For this review, take the finished solid that the model builds, in its own axes (mm). Round coordinates to 2 decimals unless told otherwise and drop trailing zeros. Order: outer loops, then holes, each group sorted by start corner. A loop starts at its lowest first (then second) coordinate and runs counter-clockwise, first axis right, second up. Notation, with made-up numbers: M 23.5,58 L 76.5,58 A17 ccw 76.5,73 Z; hole C 64,28.5 d10. An arc over 180 degrees is marked long. Put each result on its own line as item: value.
from build123d import *

# Parameters (mm, degrees)
TABAN_FLAN_4_DEPTH     = 380
KES_EKSTR_ZYON11_DEPTH = 10


# Sheet-metal steps are written as plain solids
with BuildPart() as part:
    # Çizim18 → Taban-Flanş4 (new body)
    with BuildSketch(Plane(origin=(0, 0, 0), x_dir=(0, 0, -1), z_dir=(1, 0, 0))):
        with BuildLine():
            Line((-5.5, 17.5), (-5.5, 13.2366))
            ThreePointArc((-5.5, 13.2366), (-5.284254855, 12.715745145), (-4.7634, 12.5))
            Line((-4.7634, 12.5), (-2.7366, 12.5))
            ThreePointArc((-2.7366, 12.5), (-0.801531583, 11.698468417), (0, 9.7634))
            Line((0, 9.7634), (0, -9.7634))
            ThreePointArc((0, -9.7634), (-0.801531583, -11.698468417), (-2.7366, -12.5))
            Line((-2.7366, -12.5), (-4.7634, -12.5))
            ThreePointArc((-4.7634, -12.5), (-5.284254855, -12.715745145), (-5.5, -13.2366))
            Line((-5.5, -13.2366), (-5.5, -17.5))
            Line((-5.5, -17.5), (-7.5, -17.5))
            Line((-7.5, -17.5), (-7.5, -13.2366))
            ThreePointArc((-7.5, -13.2366), (-6.698468417, -11.301531583), (-4.7634, -10.5))
            Line((-4.7634, -10.5), (-2.7366, -10.5))
            ThreePointArc((-2.7366, -10.5), (-2.215745145, -10.284254855), (-2, -9.7634))
            Line((-2, -9.7634), (-2, 9.7634))
            ThreePointArc((-2, 9.7634), (-2.215745145, 10.284254855), (-2.7366, 10.5))
            Line((-2.7366, 10.5), (-4.7634, 10.5))
            ThreePointArc((-4.7634, 10.5), (-6.698468417, 11.301531583), (-7.5, 13.2366))
            Line((-7.5, 13.2366), (-7.5, 17.5))
            Line((-7.5, 17.5), (-5.5, 17.5))
        make_face()
    extrude(amount=TABAN_FLAN_4_DEPTH)

    # Çizim21 → Kes-Ekstrüzyon11 (cut)
    with BuildSketch(Plane.XY.offset(2)):
        with BuildLine():
            Line((8.1, 3.1), (16.9, 3.1))
            ThreePointArc((16.9, 3.1), (20, 0), (16.9, -3.1))
            Line((16.9, -3.1), (8.1, -3.1))
            ThreePointArc((8.1, -3.1), (5, 0), (8.1, 3.1))
        make_face()
        with BuildLine():
            Line((28.1, 3.1), (36.9, 3.1))
            ThreePointArc((36.9, 3.1), (40, 0), (36.9, -3.1))
            Line((36.9, -3.1), (28.1, -3.1))
            ThreePointArc((28.1, -3.1), (25, 0), (28.1, 3.1))
        make_face()
        with BuildLine():
            Line((48.1, 3.1), (56.9, 3.1))
            ThreePointArc((56.9, 3.1), (60, 0), (56.9, -3.1))
            Line((56.9, -3.1), (48.1, -3.1))
            ThreePointArc((48.1, -3.1), (45, 0), (48.1, 3.1))
        make_face()
        with BuildLine():
            Line((68.1, 3.1), (76.9, 3.1))
            ThreePointArc((76.9, 3.1), (80, 0), (76.9, -3.1))
            Line((76.9, -3.1), (68.1, -3.1))
            ThreePointArc((68.1, -3.1), (65, 0), (68.1, 3.1))
        make_face()
        with BuildLine():
            Line((88.1, 3.1), (96.9, 3.1))
            ThreePointArc((96.9, 3.1), (100, 0), (96.9, -3.1))
            Line((96.9, -3.1), (88.1, -3.1))
            ThreePointArc((88.1, -3.1), (85, 0), (88.1, 3.1))
        make_face()
        with BuildLine():
            Line((108.1, 3.1), (116.9, 3.1))
            ThreePointArc((116.9, 3.1), (120, 0), (116.9, -3.1))
            Line((116.9, -3.1), (108.1, -3.1))
            ThreePointArc((108.1, -3.1), (105, 0), (108.1, 3.1))
        make_face()
        with BuildLine():
            Line((128.1, 3.1), (136.9, 3.1))
            ThreePointArc((136.9, 3.1), (140, 0), (136.9, -3.1))
            Line((136.9, -3.1), (128.1, -3.1))
            ThreePointArc((128.1, -3.1), (125, 0), (128.1, 3.1))
        make_face()
        with BuildLine():
            Line((148.1, 3.1), (156.9, 3.1))
            ThreePointArc((156.9, 3.1), (160, 0), (156.9, -3.1))
            Line((156.9, -3.1), (148.1, -3.1))
            ThreePointArc((148.1, -3.1), (145, 0), (148.1, 3.1))
        make_face()
        with BuildLine():
            Line((168.1, 3.1), (176.9, 3.1))
            ThreePointArc((176.9, 3.1), (180, 0), (176.9, -3.1))
            Line((176.9, -3.1), (168.1, -3.1))
            ThreePointArc((168.1, -3.1), (165, 0), (168.1, 3.1))
        make_face()
        with BuildLine():
            Line((188.1, 3.1), (196.9, 3.1))
            ThreePointArc((196.9, 3.1), (200, 0), (196.9, -3.1))
            Line((196.9, -3.1), (188.1, -3.1))
            ThreePointArc((188.1, -3.1), (185, 0), (188.1, 3.1))
        make_face()
        with BuildLine():
            Line((208.1, 3.1), (216.9, 3.1))
            ThreePointArc((216.9, 3.1), (220, 0), (216.9, -3.1))
            Line((216.9, -3.1), (208.1, -3.1))
            ThreePointArc((208.1, -3.1), (205, 0), (208.1, 3.1))
        make_face()
        with BuildLine():
            Line((228.1, 3.1), (236.9, 3.1))
            ThreePointArc((236.9, 3.1), (240, 0), (236.9, -3.1))
            Line((236.9, -3.1), (228.1, -3.1))
            ThreePointArc((228.1, -3.1), (225, 0), (228.1, 3.1))
        make_face()
        with BuildLine():
            Line((248.1, 3.1), (256.9, 3.1))
            ThreePointArc((256.9, 3.1), (260, 0), (256.9, -3.1))
            Line((256.9, -3.1), (248.1, -3.1))
            ThreePointArc((248.1, -3.1), (245, 0), (248.1, 3.1))
        make_face()
        with BuildLine():
            Line((268.1, 3.1), (276.9, 3.1))
            ThreePointArc((276.9, 3.1), (280, 0), (276.9, -3.1))
            Line((276.9, -3.1), (268.1, -3.1))
            ThreePointArc((268.1, -3.1), (265, 0), (268.1, 3.1))
        make_face()
        with BuildLine():
            Line((288.1, 3.1), (296.9, 3.1))
            ThreePointArc((296.9, 3.1), (300, 0), (296.9, -3.1))
            Line((296.9, -3.1), (288.1, -3.1))
            ThreePointArc((288.1, -3.1), (285, 0), (288.1, 3.1))
        make_face()
        with BuildLine():
            Line((308.1, 3.1), (316.9, 3.1))
            ThreePointArc((316.9, 3.1), (320, 0), (316.9, -3.1))
            Line((316.9, -3.1), (308.1, -3.1))
            ThreePointArc((308.1, -3.1), (305, 0), (308.1, 3.1))
        make_face()
        with BuildLine():
            Line((328.1, 3.1), (336.9, 3.1))
            ThreePointArc((336.9, 3.1), (340, 0), (336.9, -3.1))
            Line((336.9, -3.1), (328.1, -3.1))
            ThreePointArc((328.1, -3.1), (325, 0), (328.1, 3.1))
        make_face()
        with BuildLine():
            Line((348.1, 3.1), (356.9, 3.1))
            ThreePointArc((356.9, 3.1), (360, 0), (356.9, -3.1))
            Line((356.9, -3.1), (348.1, -3.1))
            ThreePointArc((348.1, -3.1), (345, 0), (348.1, 3.1))
        make_face()
    extrude(amount=-KES_EKSTR_ZYON11_DEPTH, mode=Mode.SUBTRACT)


solid = part.part
(1) Draft analysis for pull direction Y (two halves, no side actions). For faces 1 (the face through (187, 4, 0)), 2 (the face through (187, -4, 2)), state which applies: released by +Y, released by -Y, zero draft, split by the parting line, or undercut.
A:
face 1: zero draft
face 2: undercut
(2) Add section B-B on y = 0. State how many separate pieces and enclosed holes the cut face has, then the cut area to 3 significant figures.
A:
separate pieces: 19
enclosed holes: 0
area: 220 mm2
(3) Insertion check: pin 1 Ø1 at (x, z) = (234.5, 0.5) entering from +Y; pin 2 Ø1.6 at (x, z) = (273, 0.5) entering from +Y; pin 3 Ø2 at (x, z) = (112.5, 0.5) entering from +Y. Each pin has a flat end and moves straight along its axis. Give the tip position at first contact, or say it passes through.
A:
pin 1: stops at y = 11.88
pin 2: stops at y = 12.09
pin 3: stops at y = 12.2
(4) Add section A-A on x = 152.5. Give the boundary of the cut face in (y, z).
A:
outline: M -17.5,5.5 L -13.24,5.5 A0.74 cw -12.5,4.76 L -12.5,2.74 A2.74 ccw -9.76,0 L -3.1,0 L -3.1,2 L -9.76,2 A0.74 cw -10.5,2.74 L -10.5,4.76 A2.74 ccw -13.24,7.5 L -17.5,7.5 Z; M 3.1,0 L 9.76,0 A2.74 ccw 12.5,2.74 L 12.5,4.76 A0.74 cw 13.24,5.5 L 17.5,5.5 L 17.5,7.5 L 13.24,7.5 A2.74 ccw 10.5,4.76 L 10.5,2.74 A0.74 cw 9.76,2 L 3.1,2 Z
(5) To check wall thickness, follow L1, parallel to Y at x = 250, z = 3; L2, parallel to Y at x = 220, z = 7.25; L3, parallel to Z at x = 254.5, y = -13. State the ranges of each line that lie inside material, in increasing order.
A:
L1: y = -12.5 to -10.5, 10.5 to 12.5
L2: y = -17.5 to -12.09, 12.09 to 17.5
L3: z = 5.46 to 7.49
